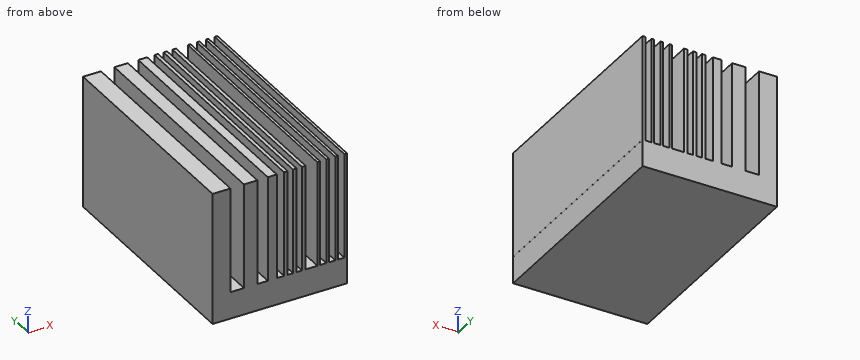
from build123d import *

# Parameters (mm, degrees)
F0_W     = 5.08
F0_H     = 25.4
F0_W_2   = 2.54
F0_W_3   = 3.81
F1_DEPTH = 40
F3_W     = 2
F3_H     = 11.758205078
F3_W_2   = 1.5
F3_W_3   = 1
F3_W_4   = 0.3
F3_W_5   = 0.4
F4_DEPTH = 12.5


with BuildPart() as f1:
    # F0 (on Front) → F1 (new body)
    with BuildSketch(Plane.XZ):
        Polygon((-39.5374095005, -17.8057016992), (-44.6174095005, -17.8057016992), (-44.6174095005, -22.8857016992), (56.9825904995, -22.8857016992), (56.9825904995, -17.8057016992), (51.9025904995, -17.8057016992), (40.6538585508, -17.8057016992), (38.1138585508, -17.8057016992), (25.9218535846, -17.8057016992), (22.1118535846, -17.8057016992), (8.1349273361, -17.8057016992), (3.0549273361, -17.8057016992), (-17.8261825508, -17.8057016992), (-20.3661825508, -17.8057016992), (-27.4666358256, -17.8057016992), (-31.2766358256, -17.8057016992), align=None)
        with Locations((54.4425904995, -5.1057016992)):
            Rectangle(F0_W, F0_H)
        with Locations((39.3838585508, -5.1057016992)):
            Rectangle(F0_W_2, F0_H)
        with Locations((24.0168535846, -5.1057016992)):
            Rectangle(F0_W_3, F0_H)
        with Locations((5.5949273361, -5.1057016992)):
            Rectangle(F0_W, F0_H)
        with Locations((-29.3716358256, -5.1057016992)):
            Rectangle(F0_W_3, F0_H)
        with Locations((-42.0774095005, -5.1057016992)):
            Rectangle(F0_W, F0_H)
        with Locations((-19.0961825508, -5.1057016992)):
            Rectangle(F0_W_2, F0_H)
    extrude(amount=F1_DEPTH)


with BuildPart() as f4:
    # F3 (on Front) → F4 (new body, symmetric)
    with BuildSketch(Plane.XZ):
        with Locations((-14.0355701865, -5.879102539)):
            Rectangle(F3_W, F3_H)
        Polygon((-13.0355701865, -11.758205078), (-15.0355701865, -11.758205078), (-15.0355701865, -14.758205078), (-0.0355701865, -14.758205078), (-0.0355701865, -11.758205078), (-0.3316470217, -11.758205078), (-1.0316470217, -11.758205078), (-1.3316470217, -11.758205078), (-2.0316470217, -11.758205078), (-2.3316470217, -11.758205078), (-3.0316470217, -11.758205078), (-3.3316470217, -11.758205078), (-4.6532104, -11.758205078), (-5.0532104, -11.758205078), (-5.6532104, -11.758205078), (-6.0532104, -11.758205078), (-6.6532104, -11.758205078), (-7.0532104, -11.758205078), (-7.870703689, -11.758205078), (-8.870703689, -11.758205078), (-10.0352638757, -11.758205078), (-11.5352638757, -11.758205078), align=None)
        with Locations((-10.7852638757, -5.879102539)):
            Rectangle(F3_W_2, F3_H)
        Polygon((-0.3316470217, -11.758205078), (-0.0355701865, -11.758205078), (-0.0316470217, -11.758205078), (-0.0316470217, 0), (-0.3316470217, 0), align=None)
        with Locations((-8.370703689, -5.879102539)):
            Rectangle(F3_W_3, F3_H)
        with Locations((-1.1816470217, -5.879102539)):
            Rectangle(F3_W_4, F3_H)
        with Locations((-6.8532104, -5.879102539)):
            Rectangle(F3_W_5, F3_H)
        with Locations((-2.1816470217, -5.879102539)):
            Rectangle(F3_W_4, F3_H)
        with Locations((-5.8532104, -5.879102539)):
            Rectangle(F3_W_5, F3_H)
        with Locations((-3.1816470217, -5.879102539)):
            Rectangle(F3_W_4, F3_H)
        with Locations((-4.8532104, -5.879102539)):
            Rectangle(F3_W_5, F3_H)
    extrude(amount=F4_DEPTH, both=True)


solid = f4.part
Input: part model. Units: mm. Frame: model coordinates. Round coordinates to 2 decimals unless told otherwise and drop trailing zeros. Loops run counter-clockwise (first coordinate to the right, second up) from the corner with the lowest first, then second, coordinate; pieces in that order, holes last. Notation, with made-up numbers: M 71.25,47 L 130.25,47 A12 ccw 130.25,52 Z; hole C 69.25,-20 d7. An arc over 180 degrees is marked long. Answer as CSV lines item,"result". Start each with the question number.
(1) Section B-B, the plane x = -12.5. Output: boundary loops of the cut face in (y, z).
(2) Section A-A, the plane z = -5. State how many separate pieces and enclosed holes the cut face has, plus the area to 4 significant figures.
(3) Line query: line 1 (X direction, y = 0.75, z = -12.5); line 2 (Z direction, x = -1.5, y = -10.5). Output: solid intervals per line, ascending. Write a range as [from, to].
Values found:
1,outline,"M -12.5,-14.76 L 12.5,-14.76 L 12.5,-11.76 L -12.5,-11.76 Z"
2,separate pieces,"10"
2,enclosed holes,"0"
2,area,"172.5 mm²"
3,line 1,"x = [-15.04, -0.04]"
3,line 2,"z = [-14.76, -11.76]"
